Print and shaded views of the part. All mm, measured from the part's lowest x, y and z. Give positions to 0.01 mm unless a question says otherwise; leave off trailing zeros. Loops run counter-clockwise (first coordinate to the right, second up) from the corner with the lowest first, then second, coordinate; pieces in that order, holes last. Notation, with made-up numbers: M 7.25,37.5 L 59.25,37.5 A15 ccw 59.25,53.5 Z; hole C -15.75,23 d3. An arc over 180 degrees is marked long. Answer in a Markdown table with one row per item.
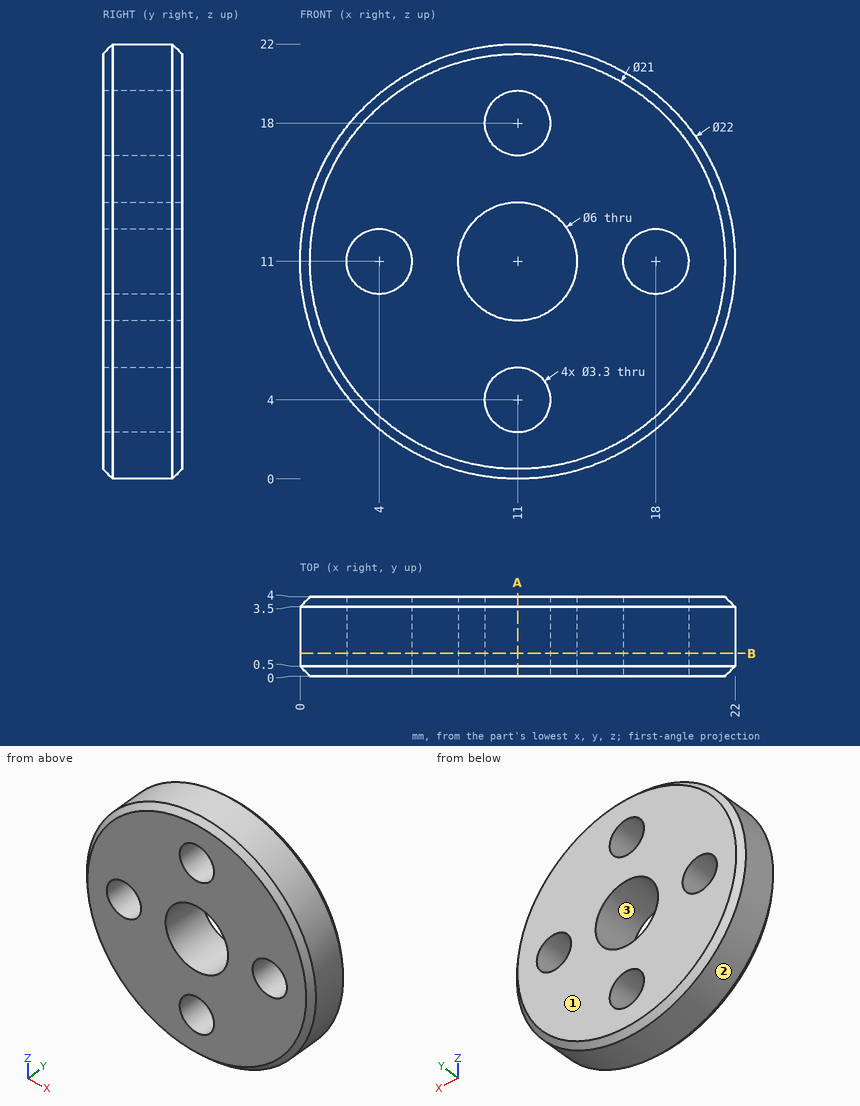
(1) Wall check: L1, parallel to X at y = 2.9, z = 11; L2, parallel to X at y = 3.7, z = 10.25; L3, parallel to Z at x = 16.5, y = 1.4. Give the ranges that are in metal, low to high.
Established:
| item | result |
|---|---|
| L1 | x = 0 to 2.35, 5.65 to 8, 14 to 16.35, 19.65 to 22 |
| L2 | x = 0.23 to 2.53, 5.47 to 8.1, 13.9 to 16.53, 19.47 to 21.77 |
| L3 | z = 1.47 to 10.31, 11.69 to 20.53 |
(2) Saw through at A-A, the plane x = 11. Give the cut face in (y, z), and give its area (3 significant figures).
Established:
| item | result |
|---|---|
| outline | M 0,0.5 L 0.5,0 L 3.5,0 L 4,0.5 L 4,2.35 L 0,2.35 Z; M 0,5.65 L 4,5.65 L 4,8 L 0,8 Z; M 0,14 L 4,14 L 4,16.35 L 0,16.35 Z; M 0,19.65 L 4,19.65 L 4,21.5 L 3.5,22 L 0.5,22 L 0,21.5 Z |
| area | 37.1 mm2 |
(3) Flat gauge pins, fed straight in: P1, Ø7, axis at x = 11, z = 11, coming from the +Y side; P2, Ø3, axis at x = 18, z = 11, coming from the -Y side. Where does each tip first touch, or does it go through?
Established:
| item | result |
|---|---|
| P1 | stops at y = 4 |
| P2 | passes through |
(4) Mould opens along X. For the marked faces 1, 2 and 3 say: pulls with the +X half, pulls with the -X half, needs draft (parallel to the pull), parting line crosses it, or undercut.
Established:
| item | result |
|---|---|
| face 1 | needs draft |
| face 2 | parting line crosses it |
| face 3 | undercut |
(5) Saw through at B-B, the plane y = 1.15. Give the cut face in (x, z).
Established:
| item | result |
|---|---|
| outline | C 11,11 d22; hole C 4,11 d3.3; hole C 11,11 d6; hole C 11,4 d3.3; hole C 11,18 d3.3; hole C 18,11 d3.3 |
